```python
from build123d import *

# Parameters (mm, degrees)
F2_W = 35
F2_H = 35
F0_W = 35
F0_H = 35


with BuildPart() as f3:
    # F2 (on offset) → F3 section 0
    with BuildSketch(Plane.XY.offset(100)):
        with Locations((-32.5, -32.5)):
            Rectangle(F2_W, F2_H)
    # F0 (on Top) → F3 section 1
    with BuildSketch(Plane.XY):
        with Locations((-32.5, -32.5)):
            Rectangle(F0_W, F0_H)
    loft()

    # F0 (on Top) → F4 section 0
    with BuildSketch(Plane.XY):
        with Locations((32.5, -32.5)):
            Rectangle(F0_W, F0_H)
    # F2 (on offset) → F4 section 1
    with BuildSketch(Plane.XY.offset(100)):
        with Locations((-32.5, -32.5)):
            Rectangle(F2_W, F2_H)
    loft()

    # F0 (on Top) → F5 section 0
    with BuildSketch(Plane.XY):
        with Locations((32.5, -32.5)):
            Rectangle(F0_W, F0_H)
    # F2 (on offset) → F5 section 1
    with BuildSketch(Plane.XY.offset(100)):
        with Locations((32.5, -32.5)):
            Rectangle(F2_W, F2_H)
    loft()



with BuildPart() as f6:
    # F0 (on Top) → F6 section 0
    with BuildSketch(Plane.XY):
        with Locations((32.5, 32.5)):
            Rectangle(F0_W, F0_H)
    # F2 (on offset) → F6 section 1
    with BuildSketch(Plane.XY.offset(100)):
        with Locations((32.5, 32.5)):
            Rectangle(F2_W, F2_H)
    loft()


with BuildPart() as f3_1:
    add(f3.part)

    add(f6.part)  # F7 merges F6
    # F0 (on Top) → F7 section 0
    with BuildSketch(Plane.XY):
        with Locations((32.5, 32.5)):
            Rectangle(F0_W, F0_H)
    # F2 (on offset) → F7 section 1
    with BuildSketch(Plane.XY.offset(100)):
        with Locations((32.5, -32.5)):
            Rectangle(F2_W, F2_H)
    loft()

    # F2 (on offset) → F8 section 0
    with BuildSketch(Plane.XY.offset(100)):
        with Locations((32.5, 32.5)):
            Rectangle(F2_W, F2_H)
    # F0 (on Top) → F8 section 1
    with BuildSketch(Plane.XY):
        with Locations((-32.5, 32.5)):
            Rectangle(F0_W, F0_H)
    loft()

    # F2 (on offset) → F9 section 0
    with BuildSketch(Plane.XY.offset(100)):
        with Locations((-32.5, 32.5)):
            Rectangle(F2_W, F2_H)
    # F0 (on Top) → F9 section 1
    with BuildSketch(Plane.XY):
        with Locations((-32.5, 32.5)):
            Rectangle(F0_W, F0_H)
    loft()

    # F2 (on offset) → F10 section 0
    with BuildSketch(Plane.XY.offset(100)):
        with Locations((-32.5, 32.5)):
            Rectangle(F2_W, F2_H)
    # F0 (on Top) → F10 section 1
    with BuildSketch(Plane.XY):
        with Locations((-32.5, -32.5)):
            Rectangle(F0_W, F0_H)
    loft()


solid = f3_1.part
```
Source: CAD feature listing. Evaluate the final solid. Frame: model axes, mm. A direction names the side the tool comes from. Coordinates: 2 decimals unless noted, no trailing zeros. Write each loop counter-clockwise with the first axis right and the second up, starting at its lowest first coordinate (ties: lowest second). Pieces come first, ordered by that corner, then holes. Notation, with made-up numbers: (-3, -12.75) -> (39, -12.75) arc R20 ccw to (39, 11.25) -> close; hole circle Ø5 at (67.25, -10). An arc over 180 degrees is marked (long way). Return JSON: item names as keys, results as strings. Group by question number.
1) Contact query for flat-ended pins moving along their axis: P1, Ø3, axis at y = 11.5, z = 22.5, coming from the -X side; P2, Ø12, axis at x = -13.5, y = 30, coming from the -Z side; P3, Ø4, axis at x = -14, y = 11, coming from the -Z side; P4, Ø2, axis at x = 22, y = 9, coming from the -Z side. Output: stop coordinate, or through.
2) Set-up query: faces 1 (the face through (-1, 15, 49)), 2 (the face through (-0.21, -32.26, 23.4)), 3 (the face through (32.745, -0.21, 77.246)). Return all of +Z, -Z, +X, -X, +Y, -Y with unobstructed straight access to the full face (end or side cutting, diameter ignored); none if empty.
3) Section query A-A, the plane z = 12. Return loops of the section in (x, y), plus the area to 3 significant figures.
4) Section query B-B, the plane y = 13. Return loops of the section in (x, z).
5) Ray query, line 1 along X through (y, z) = (13.5, 53); line 2 along X through (y, z) = (8, 66). Return the intervals inside material, ascending.
6) Section query C-C, the plane x = -25.5. Return loops of the section in (y, z), plus the area to 3 significant figures.
7) Mould query, pull axis Y, two halves, no side actions, for faces 4 (the face through (-32.255, -0.21, 22.754)), 5 (the face through (1, 50, 49)), 6 (the face through (-50, 0, 49)), 7 (the face through (-1, -50, 50)). Classes: +Y half, -Y half, draft (parallel to the pull), parting line (faces both ways), or undercut.
8) Section query D-D, the plane x = -1. Return loops of the section in (y, z).
From the geometry:
{
 "1": {"P1": "x = 15", "P2": "z = 0", "P3": "z = 37.34", "P4": "z = 7.69"},
 "2": {"face 1": "none", "face 2": "-Z, -Y", "face 3": "+Z, +X"},
 "3": {"outline": "(-50, -50) -> (-15, -50) -> (-15, -7.2) -> (-50, -7.2) -> close; (-50, 15) -> (-7.2, 15) -> (-7.2, 50) -> (-50, 50) -> close; (7.2, -50) -> (50, -50) -> (50, -15) -> (7.2, -15) -> close; (15, 7.2) -> (50, 7.2) -> (50, 50) -> (15, 50) -> close", "area": "5,990 mm²"},
 "4": {"outline": "(-50, 43.08) -> (-15, 43.08) -> (-15, 96.92) -> (-50, 96.92) -> close; (15, 3.08) -> (50, 3.08) -> (50, 56.92) -> (15, 56.92) -> close"},
 "5": {"line 1": "-50 to -15, 15 to 50", "line 2": "-50 to -15"},
 "6": {"outline": "(-50, 0) -> (-15, 0) -> (15, 46.15) -> (15, 0) -> (50, 0) -> (50, 100) -> (15, 100) -> (-15, 53.85) -> (-15, 100) -> (-50, 100) -> close", "area": "8,620 mm²"},
 "7": {"face 4": "undercut", "face 5": "+Y half", "face 6": "draft", "face 7": "-Y half"},
 "8": {"outline": "(-50, 24.62) -> (-15, 24.62) -> (-15, 78.46) -> (-50, 78.46) -> close; (15, 21.54) -> (50, 21.54) -> (50, 75.38) -> (15, 75.38) -> close"}
}
